from build123d import *

# Parameters (mm, degrees)
SKETCH_1_W      = 11.9
SKETCH_1_H      = 23.7
EXTRUDE_1_DEPTH = 16.4
SKETCH_2_R      = 1
EXTRUDE_2_DEPTH = 1.5
SKETCH_3_W      = 11.9
SKETCH_3_H      = 23.7
EXTRUDE_3_DEPTH = 4.1
EXTRUDE_4_DEPTH = 4.6
SKETCH_5_R      = 2.5
SKETCH_5_R_2    = 1
EXTRUDE_5_DEPTH = 3.2


with BuildPart() as part:
    # 草图1 → 凸台-拉伸1 (new body)
    with BuildSketch(Plane(origin=(0, 0, 0), x_dir=(1, 0, 0), z_dir=(0, 1, 0))):
        Rectangle(SKETCH_1_W, SKETCH_1_H)
    extrude(amount=EXTRUDE_1_DEPTH)

    # 草图2 → 凸台-拉伸2 (add)
    with BuildSketch(Plane(origin=(0, 16.4, 0), x_dir=(1, 0, 0), z_dir=(0, 1, 0))):
        Polygon((-5.95, 11.85), (-4.95, 15.85), (4.95, 15.85), (5.95, 11.85), (5.95, -11.85), (4.95, -15.85), (-4.95, -15.85), (-5.95, -11.85), align=None)
        with Locations(Location((0, 13.85, 0), (0, 0, 270))):
            Circle(SKETCH_2_R, mode=Mode.SUBTRACT)
        with Locations(Location((0, -13.85, 0), (0, 0, 270))):
            Circle(SKETCH_2_R, mode=Mode.SUBTRACT)
    extrude(amount=EXTRUDE_2_DEPTH)

    # 草图3 → 凸台-拉伸3 (add)
    with BuildSketch(Plane(origin=(0, 17.9, 0), x_dir=(1, 0, 0), z_dir=(0, 1, 0))):
        Rectangle(SKETCH_3_W, SKETCH_3_H)
    extrude(amount=EXTRUDE_3_DEPTH)

    # 草图4 → 凸台-拉伸4 (add)
    with BuildSketch(Plane(origin=(0, 22, 0), x_dir=(1, 0, 0), z_dir=(0, 1, 0))):
        with BuildLine():
            Line((-5.95, 7.620627924), (-5.95, 3.479372076))
            ThreePointArc((-5.95, 3.479372076), (0, -0.75), (5.95, 3.479372076))
            Line((5.95, 3.479372076), (5.95, 7.620627924))
            ThreePointArc((5.95, 7.620627924), (0, 11.85), (-5.95, 7.620627924))
        make_face()
    extrude(amount=EXTRUDE_4_DEPTH)

    # 草图5 → 凸台-拉伸5 (add)
    with BuildSketch(Plane(origin=(0, 26.6, 0), x_dir=(1, 0, 0), z_dir=(0, 1, 0))):
        with Locations(Location((0, 5.55, 0), (0, 0, 90))):
            Circle(SKETCH_5_R)
        with Locations(Location((0, 5.55, 0), (0, 0, 90))):
            Circle(SKETCH_5_R_2, mode=Mode.SUBTRACT)
    extrude(amount=EXTRUDE_5_DEPTH)


solid = part.part
Geometry: final body of the model. Coordinates: model frame, mm. A direction names the side the tool comes from. Give positions to 0.01 mm unless a question says otherwise; leave off trailing zeros. Write each loop counter-clockwise with the first axis right and the second up, starting at its lowest first coordinate (ties: lowest second). Pieces come first, ordered by that corner, then holes. Notation, with made-up numbers: (-17.75, -29) -> (32.25, -29) arc R32 cw to (32.25, 9) -> close; hole circle Ø2 at (18, 74). An arc over 180 degrees is marked (long way). Answer in a Markdown table with one row per item.
(1) Section query A-A on z = 13.85. Return loops of the section in (x, y).
Answers below:
| item | result |
|---|---|
| outline | (-5.45, 16.4) -> (-1, 16.4) -> (-1, 17.9) -> (-5.45, 17.9) -> close; (1, 16.4) -> (5.45, 16.4) -> (5.45, 17.9) -> (1, 17.9) -> close |
(2) Section query D-D on x = -4.5. Return loops of the section in (y, z).
Answers below:
| item | result |
|---|---|
| outline | (0, -11.85) -> (16.4, -11.85) -> (16.4, -15.85) -> (17.9, -15.85) -> (17.9, -11.85) -> (22, -11.85) -> (22, -9.96) -> (26.6, -9.96) -> (26.6, -1.14) -> (22, -1.14) -> (22, 11.85) -> (17.9, 11.85) -> (17.9, 15.85) -> (16.4, 15.85) -> (16.4, 11.85) -> (0, 11.85) -> close |
(3) Ray query, line 1 along X through (y, z) = (28.6, -5.55); line 2 along Y through (x, z) = (-4.25, -6); line 3 along Y through (x, z) = (-2.75, 2). Return the intervals inside material, ascending. Write a range as [from, to].
Answers below:
| item | result |
|---|---|
| line 1 | [-2.5, -1], [1, 2.5] |
| line 2 | [0, 26.6] |
| line 3 | [0, 22] |
(4) Pin query (flat end, axial travel): pin 1 (3 mm diameter, centred on x = 0, z = -13.85, fed in from +Y); pin 2 (2 mm diameter, centred on x = 2.5, z = -13, fed in from -Y); pin 3 (1.5 mm diameter, centred on x = -1, z = 11.5, fed in from -Y); pin 4 (4.5 mm diameter, centred on x = -2, z = 13.5, fed in from +Y). Return the tip coordinate at first contact, or that it passes through.
Answers below:
| item | result |
|---|---|
| pin 1 | y = 17.9 |
| pin 2 | y = 16.4 |
| pin 3 | y = 0 |
| pin 4 | y = 22 |
(5) Draft query along Z for faces 1 (the cylindrical face through (-0.751, 28.178, -7.935)), 2 (the cylindrical face through (-0.04, 28.18, -4.55)), 3 (the flat face through (0, 8, -11.85)). Return one class per face: +Z half, -Z half, draft (parallel to the pull), parting line (faces both ways), or undercut.
Answers below:
| item | result |
|---|---|
| face 1 | parting line |
| face 2 | undercut |
| face 3 | -Z half |
(6) Section query C-C on z = -5.55. Return loops of the section in (x, y), then the cut area to 3 significant figures.
Answers below:
| item | result |
|---|---|
| outline | (-5.95, 0) -> (5.95, 0) -> (5.95, 26.6) -> (2.5, 26.6) -> (2.5, 29.8) -> (1, 29.8) -> (1, 26.6) -> (-1, 26.6) -> (-1, 29.8) -> (-2.5, 29.8) -> (-2.5, 26.6) -> (-5.95, 26.6) -> close |
| area | 326 mm^2 |
(7) Set-up query: faces 4 (the flat face through (-5, 22, -11)), 5 (the cylindrical face through (-0.11, 24.27, 0.75)), 6 (the flat face through (-1.2, 17.9, -13.9)), 7 (the flat face through (-1.2, 16.4, 13.8)), 8 (the flat face through (0, 20, 11.85)). Return all of +Z, -Z, +X, -X, +Y, -Y with unobstructed straight access to the full face (end or side cutting, diameter ignored); none if empty.
Answers below:
| item | result |
|---|---|
| face 4 | -Z, -X, +Y |
| face 5 | +Z, +Y |
| face 6 | -Z, +X, -X, +Y |
| face 7 | +Z, +X, -X, -Y |
| face 8 | +Z, +X, -X, +Y |
(8) Section query B-B on y = 17.25. Return loops of the section in (x, z).
Answers below:
| item | result |
|---|---|
| outline | (-5.95, -11.85) -> (-4.95, -15.85) -> (4.95, -15.85) -> (5.95, -11.85) -> (5.95, 11.85) -> (4.95, 15.85) -> (-4.95, 15.85) -> (-5.95, 11.85) -> close; hole circle Ø2 at (0, -13.85); hole circle Ø2 at (0, 13.85) |
